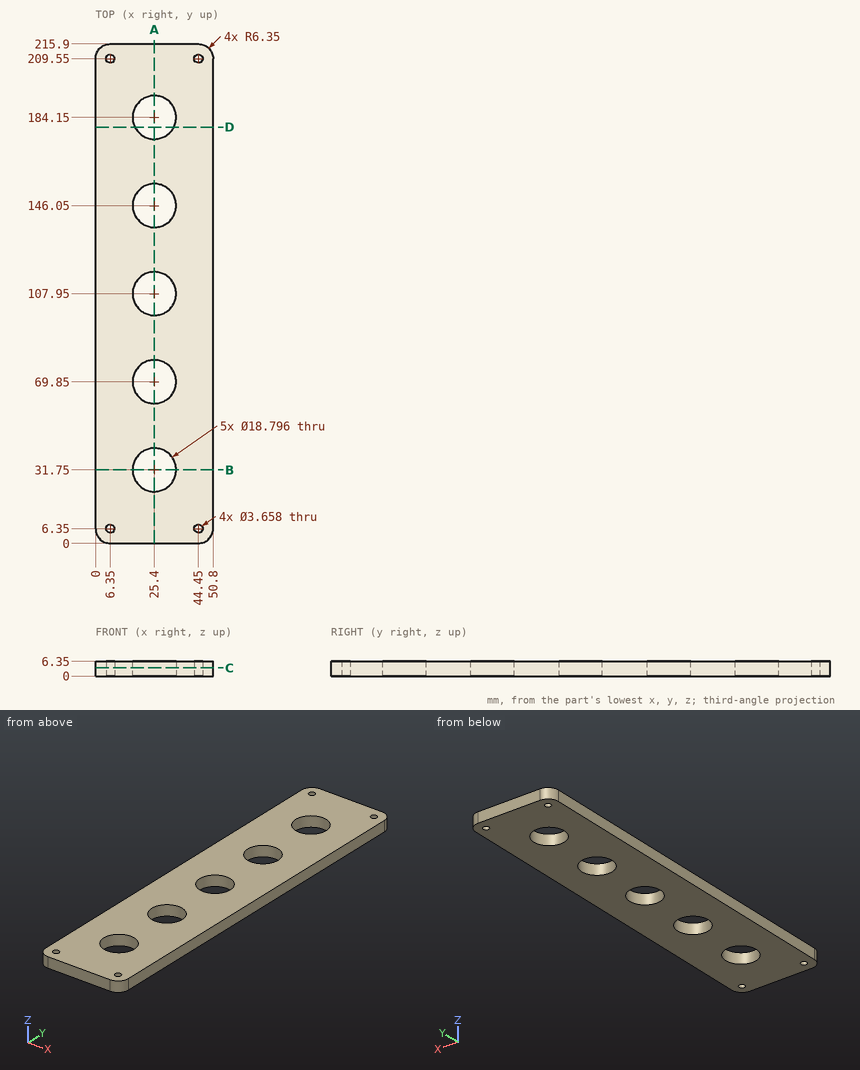
Geometry check sheet. Reference: drawing and pictorial views, mm from the part's lowest x, y, z. Give positions to 0.01 mm unless a question says otherwise; leave off trailing zeros. Loops run counter-clockwise (first coordinate to the right, second up) from the corner with the lowest first, then second, coordinate; pieces in that order, holes last. Notation, with made-up numbers: M 89.25,-19 L 101.25,-19 A31 cw 101.25,12 Z; hole C 73.5,19.25 d7. An arc over 180 degrees is marked long. One line per question, with ' | ' between items.
Item 1: Section check A-A, the plane x = 25.4. Record the cut outline in (y, z).
Completed:
outline: M 0,0 L 22.35,0 L 22.35,6.35 L 0,6.35 Z; M 41.15,0 L 60.45,0 L 60.45,6.35 L 41.15,6.35 Z; M 79.25,0 L 98.55,0 L 98.55,6.35 L 79.25,6.35 Z; M 117.35,0 L 136.65,0 L 136.65,6.35 L 117.35,6.35 Z; M 155.45,0 L 174.75,0 L 174.75,6.35 L 155.45,6.35 Z; M 193.55,0 L 215.9,0 L 215.9,6.35 L 193.55,6.35 Z
Item 2: Thickness scan on line 1 (X direction, y = 209.55, z = 4); line 2 (Y direction, x = 44.45, z = 2.75); line 3 (Y direction, x = 25.4, z = 5). Record the ranges inside material, lowest first. Write a range as [from, to].
Completed:
line 1: x = [0, 4.52], [8.18, 42.62], [46.28, 50.8] | line 2: y = [0, 4.52], [8.18, 207.72], [211.38, 215.9] | line 3: y = [0, 22.35], [41.15, 60.45], [79.25, 98.55], [117.35, 136.65], [155.45, 174.75], [193.55, 215.9]
Item 3: Section check C-C, the plane z = 3.5. State how many separate pieces and enclosed holes the cut face has, plus the area to 3 significant figures.
Completed:
separate pieces: 1 | enclosed holes: 9 | area: 9,500 mm^2
Item 4: Section check D-D, the plane y = 180. Record the cut outline in (x, z).
Completed:
outline: M 0,0 L 16.97,0 L 16.97,6.35 L 0,6.35 Z; M 33.83,0 L 50.8,0 L 50.8,6.35 L 33.83,6.35 Z
Item 5: Depth check by flat-ended pin: P1, Ø3.5, axis at x = 6.35, y = 6.35, coming from the -Z side. Enter the tip coordinate at first touch or a pass-through.
Completed:
P1: passes through
Item 6: Section check B-B, the plane y = 31.75. Record the cut outline in (x, z).
Completed:
outline: M 0,0 L 16,0 L 16,6.35 L 0,6.35 Z; M 34.8,0 L 50.8,0 L 50.8,6.35 L 34.8,6.35 Z
